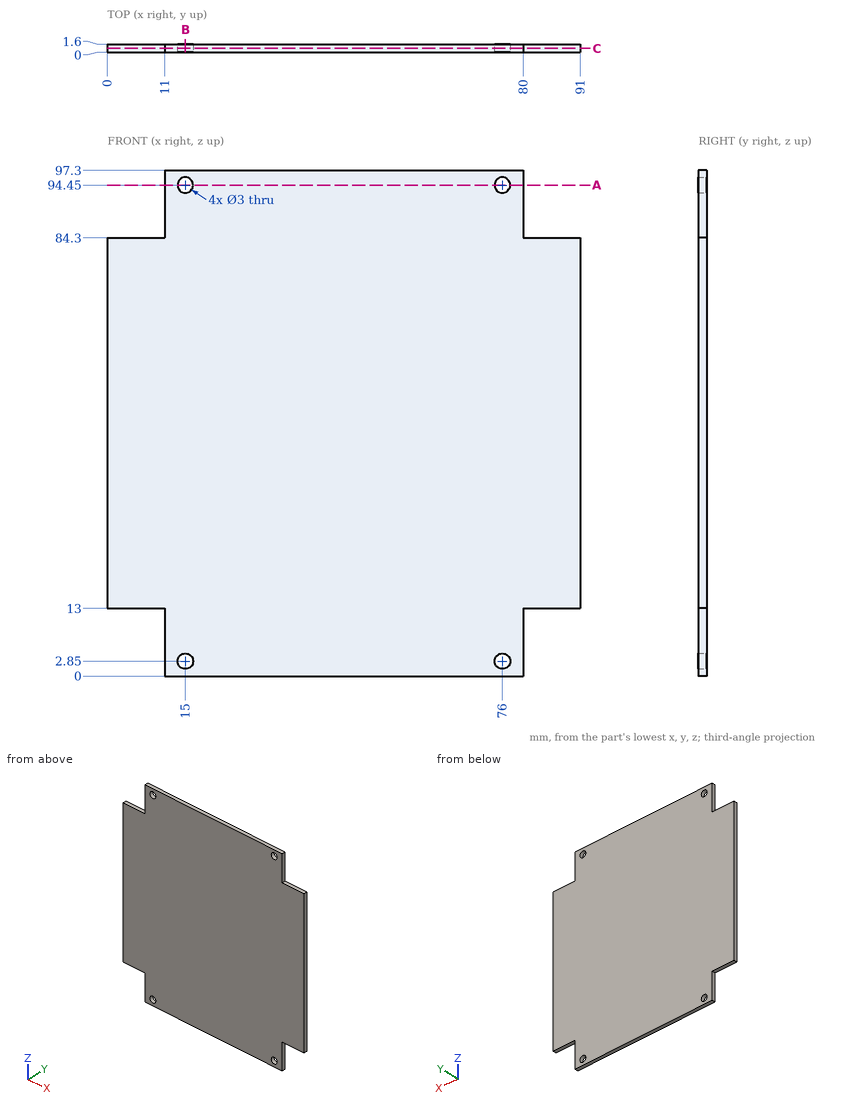
Verification items for this drawing (mm, ordinates from the low corner). Coordinates: 2 decimals unless noted, no trailing zeros. Order: outer loops, then holes, each group sorted by start corner. A loop starts at its lowest first (then second) coordinate and runs counter-clockwise, first axis right, second up.
Q1. Sectioned sample at C-C on y = 0.75. Record the cut outline in (x, z).
Reply:
outline: (0, 13) - (11, 13) - (11, 0) - (80, 0) - (80, 13) - (91, 13) - (91, 84.3) - (80, 84.3) - (80, 97.3) - (11, 97.3) - (11, 84.3) - (0, 84.3) - close; hole circle Ø3 at (15, 2.85); hole circle Ø3 at (15, 94.45); hole circle Ø3 at (76, 2.85); hole circle Ø3 at (76, 94.45)
Q2. Depth check by flat-ended pin: pin 1 Ø0.8 at (y, z) = (1, 4) entering from -X; pin 2 Ø0.8 at (x, y) = (6, 0.5) entering from -Z; pin 3 Ø0.5 at (y, z) = (1, 90.5) entering from +X. Enter the tip coordinate at first touch or a pass-through.
Reply:
pin 1: stops at x = 11
pin 2: stops at z = 13
pin 3: stops at x = 80
Q3. Sectioned sample at A-A on z = 94.45. Record the cut outline in (x, y), and give its area (3 significant figures).
Reply:
outline: (11, 0) - (13.5, 0) - (13.5, 1.6) - (11, 1.6) - close; (16.5, 0) - (74.5, 0) - (74.5, 1.6) - (16.5, 1.6) - close; (77.5, 0) - (80, 0) - (80, 1.6) - (77.5, 1.6) - close
area: 101 mm2
Q4. Thickness scan on probe 1 along Z at (x, y) = (76, 0.75); probe 2 along X at (y, z) = (1.15, 94.45); probe 3 along X at (y, z) = (0.45, 88.5). Record the ranges inside material, lowest first.
Reply:
probe 1: z = 0 to 1.35, 4.35 to 92.95, 95.95 to 97.3
probe 2: x = 11 to 13.5, 16.5 to 74.5, 77.5 to 80
probe 3: x = 11 to 80
Q5. Sectioned sample at B-B on x = 15. Record the cut outline in (y, z).
Reply:
outline: (0, 0) - (1.6, 0) - (1.6, 1.35) - (0, 1.35) - close; (0, 4.35) - (1.6, 4.35) - (1.6, 92.95) - (0, 92.95) - close; (0, 95.95) - (1.6, 95.95) - (1.6, 97.3) - (0, 97.3) - close
